Read the model definition and answer for the solid it produces. Units are mm, in the model's axes. Face numbers are marked on the shaded views. A direction names the side the tool comes from. Coordinates: 2 decimals unless noted, no trailing zeros. Order: outer loops, then holes, each group sorted by start corner. A loop starts at its lowest first (then second) coordinate and runs counter-clockwise, first axis right, second up.
```python
from build123d import *

# Parameters (mm, degrees)
BOSS_EXTRUDE1_DEPTH      = 8
BOSS_EXTRUDE1_DEPTH_BACK = 2
SKETCH2_W                = 38
SKETCH2_H                = 112.5
CUT_EXTRUDE1_START       = -2
CUT_EXTRUDE1_DEPTH       = 7
SKETCH3_3_R              = 2
CUT_EXTRUDE2_DEPTH       = 60.908784832
LPATTERN1_COUNT          = 2
LPATTERN1_PITCH          = 45
LPATTERN1_COL_COUNT      = 2
LPATTERN1_COL_PITCH      = 45
FILLET1_R                = 3
CHAMFER1_START           = 75
CHAMFER1_DEPTH           = 12
CUT_EXTRUDE3_DEPTH       = 105.74678766
CUT_EXTRUDE3_DEPTH_BACK  = 105.74678766
SKETCH1_R                = 78.2955


with BuildPart() as part:
    # Sketch2 → Boss-Extrude1 (new, two sides: drawn at the far end of the back side and taken through both)
    with BuildSketch(Plane(origin=(78.295, 0, 0), x_dir=(0, 0, -1), z_dir=(1, 0, 0)).offset(-BOSS_EXTRUDE1_DEPTH_BACK)):
        Rectangle(SKETCH2_W, SKETCH2_H)
    extrude(amount=BOSS_EXTRUDE1_DEPTH + BOSS_EXTRUDE1_DEPTH_BACK)

    # Sketch3 → Cut-Extrude1 (cut)
    with BuildSketch(Plane(origin=(78.295, 0, 0), x_dir=(0, 0, -1), z_dir=(1, 0, 0)).offset(CUT_EXTRUDE1_START)):
        with BuildLine():
            Line((-11.15, -7.65), (11.15, -7.65))
            ThreePointArc((11.15, -7.65), (13.978427125, -6.478427125), (15.15, -3.65))
            Line((15.15, -3.65), (15.15, 3.65))
            ThreePointArc((15.15, 3.65), (13.978427125, 6.478427125), (11.15, 7.65))
            Line((11.15, 7.65), (-11.15, 7.65))
            ThreePointArc((-11.15, 7.65), (-13.978427125, 6.478427125), (-15.15, 3.65))
            Line((-15.15, 3.65), (-15.15, -3.65))
            ThreePointArc((-15.15, -3.65), (-13.978427125, -6.478427125), (-11.15, -7.65))
        make_face()
    cut_extrude1 = extrude(amount=CUT_EXTRUDE1_DEPTH, mode=Mode.SUBTRACT)

    # Sketch3<3> → Cut-Extrude2 (cut, through all)
    with BuildSketch(Plane(origin=(78.295, 0, 0), x_dir=(0, 0, -1), z_dir=(1, 0, 0))):
        with Locations(Location((-10, 0, 0), (0, 0, 180))):
            Circle(SKETCH3_3_R)
        with Locations(Location((10, 0, 0), (0, 0, 180))):
            Circle(SKETCH3_3_R)
    cut_extrude2 = extrude(amount=CUT_EXTRUDE2_DEPTH, mode=Mode.SUBTRACT)

    # LPattern1: Cut-Extrude1, Cut-Extrude2 ×2
    with Locations(*[(0, -i * LPATTERN1_PITCH, 0) for i in range(1, LPATTERN1_COUNT)]):
        add(cut_extrude1, mode=Mode.SUBTRACT)
        add(cut_extrude2, mode=Mode.SUBTRACT)

    # LPattern1 col: Cut-Extrude1, Cut-Extrude2 ×2
    with Locations(*[(0, i * LPATTERN1_COL_PITCH, 0) for i in range(1, LPATTERN1_COL_COUNT)]):
        add(cut_extrude1, mode=Mode.SUBTRACT)
        add(cut_extrude2, mode=Mode.SUBTRACT)

    # Fillet1
    fillet1_edges = [part.edges().sort_by_distance(p)[0] for p in [
        (86.295, 0, -19),
        (86.295, 56.25, 0),
        (86.295, 0, 19),
        (86.295, -56.25, 0),
    ]]
    fillet(fillet1_edges, radius=FILLET1_R)

    # Chamfer1: read off the stored shape, not the designer's step
    # Chamfer1 outline → Chamfer1 (cut)
    with BuildSketch(Plane.YZ.offset(CHAMFER1_START)):
        Polygon((-56.25, 19), (-56.25, 13), (-50.25, 19), align=None)
        Polygon((-50.25, -19), (-56.25, -13), (-56.25, -19), align=None)
        Polygon((56.25, 19), (50.25, 19), (56.25, 13), align=None)
        Polygon((56.25, -13), (50.25, -19), (56.25, -19), align=None)
    extrude(amount=CHAMFER1_DEPTH, mode=Mode.SUBTRACT)

    # Sketch1 → Cut-Extrude3 (cut, two sides: drawn at the far end of the back side and taken through both)
    with BuildSketch(Plane(origin=(0, 0, 0), x_dir=(1, 0, 0), z_dir=(0, 1, 0)).offset(-CUT_EXTRUDE3_DEPTH_BACK)):
        Circle(SKETCH1_R)
    extrude(amount=CUT_EXTRUDE3_DEPTH + CUT_EXTRUDE3_DEPTH_BACK, mode=Mode.SUBTRACT)


solid = part.part
```
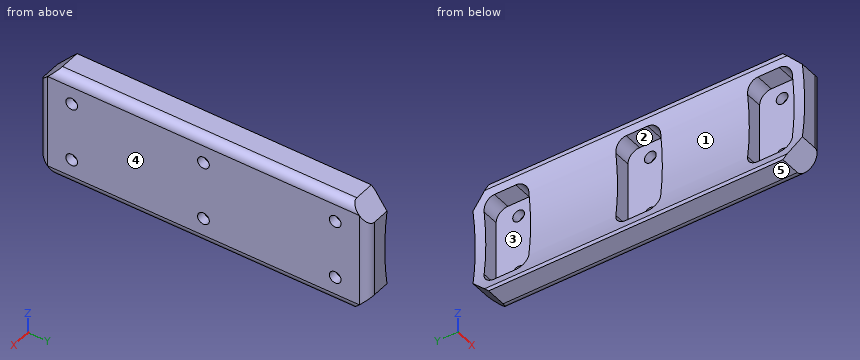
1) Straight lines are drawn through the part: line 1 (Y direction, x = 79, z = -3.5); line 2 (Z direction, x = 78.75, y = -49). For each, find the intervals that lie inside material, in ascending order.
A:
line 1: y = -56.25 to -52.65, -37.35 to -7.65, 7.65 to 37.35, 52.65 to 56.25
line 2: z = -19 to -15.13, 15.13 to 19
2) Determine the mould class of the marked faces 3, 4 and 5 for opening direction Z: pulls with the +Z half, pulls with the -Z half, needs draft (parallel to the pull), parting line crosses it, or undercut.
A:
face 3: undercut
face 4: needs draft
face 5: pulls with the -Z half
3) A cutting plane is placed at B-B, the plane y = 36. Determine the outline of the cut face in (x, z) (1 decimal).
A:
outline: (76.3, -19) - (83.3, -19) arc R3 ccw to (86.3, -16) - (86.3, 16) arc R3 ccw to (83.3, 19) - (76.3, 19) - (76.3, 17.6) arc R78.3 cw to (76.3, -17.6) - close
4) Flat-ended cylindrical pins translate along their axes: pin 1 Ø3.5 at (y, z) = (-45, -10) entering from -X; pin 2 Ø2 at (x, z) = (78.5, -15) entering from -Y; pin 3 Ø6 at (y, z) = (31, 13) entering from -X; pin 4 Ø12 at (y, z) = (44, -1.5) entering from -X (3 decimals). Find the tip coordinate at first contact, or state that the pin passes through.
A:
pin 1: passes through
pin 2: stops at y = -55.25
pin 3: stops at x = 76.64
pin 4: stops at x = 83.295
5) A cutting plane is placed at D-D, the plane z = 3. Determine the outline of the cut face in (x, y) (3 decimals).
A:
outline: (78.238, -56.25) - (83.295, -56.25) arc R3 ccw to (86.295, -53.25) - (86.295, 53.25) arc R3 ccw to (83.295, 56.25) - (78.238, 56.25) - (78.238, 52.65) - (83.295, 52.65) - (83.295, 37.35) - (78.238, 37.35) - (78.238, 7.65) - (83.295, 7.65) - (83.295, -7.65) - (78.238, -7.65) - (78.238, -37.35) - (83.295, -37.35) - (83.295, -52.65) - (78.238, -52.65) - close
6) A cutting plane is placed at A-A, the plane y = -45. State how many separate pieces and enclosed holes the cut face has, and give its area (3 significant figures).
A:
separate pieces: 3
enclosed holes: 0
area: 139 mm2
7) Which of the six approach directions +Z, -Z, +X, -X, +Y, -Y give full straight-line access (tool end or side, diameter ignored) to the marked faces 1 and 2?
A:
face 1: -X, +Y, -Y
face 2: -X
